Source: CAD feature listing. Evaluate the final solid. Frame: model axes, mm. A direction names the side the tool comes from. Coordinates: 2 decimals unless noted, no trailing zeros. Loops run counter-clockwise (first coordinate to the right, second up) from the corner with the lowest first, then second, coordinate; pieces in that order, holes last.
Autodesk Inventor part; units mm, degrees
ref_plane "YZ Plane" through (0, 0, 0) normal (1, 0, 0) x (0, 1, 0)
ref_plane "XZ Plane" through (0, 0, 0) normal (0, 1, 0) x (-1, 0, 0)
ref_plane "XY Plane" through (0, 0, 0) normal (0, 0, 1) x (1, 0, 0)
sketch "Sketch1" plane through (0, 0, 0) normal (0, 0, 1) x (1, 0, 0)
  line L0 (96, -35) -> (96, 10)
  arc A0 (88, -43) -> (96, -35) centre (88, -35) ccw
  line L1 (54, -39) -> (54, -35)
  line L2 (50, -31) -> (8, -31)
  line L3 (4, -35) -> (4, -37.1118)
  line L4 (58, -43) -> (88, -43)
  arc A1 (8, -31) -> (4, -35) centre (8, -35) ccw
  arc A2 (54, -39) -> (58, -43) centre (58, -39) ccw
  arc A3 (54, -35) -> (50, -31) centre (50, -35) ccw
  line L5 (-34, 0) -> (96, 0) construction
  line L6 (88, 18) -> (-3, 18)
  circle A4 centre (59, 12) radius 1.3
  circle A5 centre (58, -37) radius 1.3
  line L7 (4, -37.1118) -> (4, -39)
  arc A6 (0, -43) -> (4, -39) centre (0, -39) ccw
  circle A7 centre (0, -37) radius 1.3
  line L8 (58, -37) -> (0, -37) construction
  line L9 (0, 0) -> (0, 18) construction
  line L10 (0, -43) -> (-3, -43)
  line L11 (-8, -38) -> (-8, 13)
  arc A8 (-3, 18) -> (-8, 13) centre (-3, 13) ccw
  arc A9 (-8, -38) -> (-3, -43) centre (-3, -38) ccw
  arc A10 (96, 10) -> (88, 18) centre (88, 10) ccw
  circle A11 centre (0, 12) radius 1.3
  point P0 (4, -43)
  point P1 (96, 18)
  point P2 (54, -31)
  point P3 (4, -31)
  dimension "d8" = 50
  dimension "d11" = 12
  dimension "d13" = 4
  dimension "d16" = 42
  dimension "d33" = 4
  dimension "d44" = 58
  dimension "d46" = 31
  dimension "d47" = 18
  dimension "d51" = 5
  dimension "d52" = 12
  dimension "d55" = 58
  dimension "d57" = 49
  dimension "d58" = 6
  dimension "d59" = 37
  dimension "d60" = 2.6
  dimension "d61" = 8
  dimension "d62" = 8
  dimension "d64" = 4
extrude "Extrusion1" add sketch "Sketch1" along normal blind 1.56
properties part number "long_battery_mount"
Q1. Section query B-B on y = -37. Return the cut outline in (x, z).
Q2. Reachability of faces 1 (the cylindrical face through (55.203, -41.859, 0.769)), 2 (the cylindrical face through (-0.17, 10.71, 0.77)) from +Z, -Z, +X, -X, +Y, -Y: full face, straight path, thin tool, end or side. Return the list, or none.
Q3. Draft query along X for faces 3 (the flat face through (43, -12, 0)), 4 (the cylindrical face through (5.141, -32.203, 0.769)), 5 (the cylindrical face through (-7, 16, 1)). Return one class per face: released by +X, released by -X, zero draft, split by the parting line, or undercut.
Q4. Section query C-C on y = 12. Return the cut outline in (x, z).
Q5. Material intervals for line 1 along Y through (x, z) = (0, 0.45); line 2 along Y through (x, z) = (59, 0.65); line 3 along X through (y, z) = (-37.5, 0.75), sorted ascending.
Q6. First-contact query: pin 1 Ø0.8 at (y, z) = (-37.5, 1) entering from +X; pin 2 Ø1.6 at (x, y) = (58, -37) entering from +Z; pin 3 Ø10 at (x, y) = (40, -13) entering from -Z. Flat tips, straight axial feed; report the tip coordinate or a pass-through.
Q7. Section query A-A on z = 1. Return the cut outline in (x, y).
Resolved:
1. outline: (-8, 0) - (-1.3, 0) - (-1.3, 1.56) - (-8, 1.56) - close; (1.3, 0) - (4, 0) - (4, 1.56) - (1.3, 1.56) - close; (54, 0) - (56.7, 0) - (56.7, 1.56) - (54, 1.56) - close; (59.3, 0) - (95.75, 0) - (95.75, 1.56) - (59.3, 1.56) - close
2. face 1: +Z, -Z, -Y
2. face 2: +Z, -Z
3. face 3: zero draft
3. face 4: undercut
3. face 5: released by -X
4. outline: (-8, 0) - (-1.3, 0) - (-1.3, 1.56) - (-8, 1.56) - close; (1.3, 0) - (57.7, 0) - (57.7, 1.56) - (1.3, 1.56) - close; (60.3, 0) - (95.75, 0) - (95.75, 1.56) - (60.3, 1.56) - close
5. line 1: y = -43 to -38.3, -35.7 to 10.7, 13.3 to 18
5. line 2: y = -43 to -37.83, -36.17 to 10.7, 13.3 to 18
5. line 3: x = -8 to -1.2, 1.2 to 4, 54 to 56.8, 59.2 to 95.6
6. pin 1: stops at x = 95.72
6. pin 2: passes through
6. pin 3: stops at z = 0
7. outline: (-8, -38) arc R5 ccw to (-3, -43) - (0, -43) arc R4 ccw to (4, -39) - (4, -35) arc R4 cw to (8, -31) - (50, -31) arc R4 cw to (54, -35) - (54, -39) arc R4 ccw to (58, -43) - (88, -43) arc R8 ccw to (96, -35) - (96, 10) arc R8 ccw to (88, 18) - (-3, 18) arc R5 ccw to (-8, 13) - close; hole circle Ø2.6 at (0, -37); hole circle Ø2.6 at (0, 12); hole circle Ø2.6 at (58, -37); hole circle Ø2.6 at (59, 12)
